Build history of the part. All positions in model axes, mm. A direction names the side the tool comes from. Round coordinates to 2 decimals unless told otherwise and drop trailing zeros. Write each loop counter-clockwise with the first axis right and the second up, starting at its lowest first coordinate (ties: lowest second). Pieces come first, ordered by that corner, then holes. Notation, with made-up numbers: (59.5, 39.25) - (93.5, 39.25) arc R14 cw to (93.5, 46.25) - close; hole circle Ø5 at (-20, 7.25). An arc over 180 degrees is marked (long way). One line per question, with ' | ' between items.
from build123d import *

# Parameters (mm, degrees)
SKETCH1_R           = 7.5565
SKETCH1_W           = 2.54
SKETCH1_H           = 4.572
BOSS_EXTRUDE1_DEPTH = 3.175


with BuildPart() as part:
    # Sketch1 → Boss-Extrude1 (new body)
    with BuildSketch(Plane.XY):
        with BuildLine():
            Line((-8.255, 15.639992312), (76.835, 15.639992312))
            ThreePointArc((76.835, 15.639992312), (80.876115254, 13.966107566), (82.55, 9.924992312))
            Line((82.55, 9.924992312), (82.55, -9.924992312))
            ThreePointArc((82.55, -9.924992312), (80.876115254, -13.966107566), (76.835, -15.639992312))
            Line((76.835, -15.639992312), (-8.255, -15.639992312))
            ThreePointArc((-8.255, -15.639992312), (-12.296115254, -13.966107566), (-13.97, -9.924992312))
            Line((-13.97, -9.924992312), (-13.97, 9.924992312))
            ThreePointArc((-13.97, 9.924992312), (-12.296115254, 13.966107566), (-8.255, 15.639992312))
        make_face()
        Circle(SKETCH1_R, mode=Mode.SUBTRACT)
        with Locations((22.86, 0)):
            Circle(SKETCH1_R, mode=Mode.SUBTRACT)
        with Locations((45.72, 0)):
            Circle(SKETCH1_R, mode=Mode.SUBTRACT)
        with Locations((68.58, 0)):
            Circle(SKETCH1_R, mode=Mode.SUBTRACT)
        with Locations((8.636, 12.083992312)):
            Rectangle(SKETCH1_W, SKETCH1_H, mode=Mode.SUBTRACT)
        with Locations((14.224, 12.083992312)):
            Rectangle(SKETCH1_W, SKETCH1_H, mode=Mode.SUBTRACT)
        with Locations((31.496, 12.083992312)):
            Rectangle(SKETCH1_W, SKETCH1_H, mode=Mode.SUBTRACT)
        with Locations((37.084, 12.083992312)):
            Rectangle(SKETCH1_W, SKETCH1_H, mode=Mode.SUBTRACT)
        with Locations((54.356, 12.083992312)):
            Rectangle(SKETCH1_W, SKETCH1_H, mode=Mode.SUBTRACT)
        with Locations((59.944, 12.083992312)):
            Rectangle(SKETCH1_W, SKETCH1_H, mode=Mode.SUBTRACT)
        with Locations((59.944, -12.083992312)):
            Rectangle(SKETCH1_W, SKETCH1_H, mode=Mode.SUBTRACT)
        with Locations((54.356, -12.083992312)):
            Rectangle(SKETCH1_W, SKETCH1_H, mode=Mode.SUBTRACT)
        with Locations((37.084, -12.083992312)):
            Rectangle(SKETCH1_W, SKETCH1_H, mode=Mode.SUBTRACT)
        with Locations((31.496, -12.083992312)):
            Rectangle(SKETCH1_W, SKETCH1_H, mode=Mode.SUBTRACT)
        with Locations((14.224, -12.083992312)):
            Rectangle(SKETCH1_W, SKETCH1_H, mode=Mode.SUBTRACT)
        with Locations((8.636, -12.083992312)):
            Rectangle(SKETCH1_W, SKETCH1_H, mode=Mode.SUBTRACT)
    extrude(amount=BOSS_EXTRUDE1_DEPTH)


solid = part.part
Q1. Saw through at A-A, the plane x = 45.72. List the corners of the cut face in (y, z) (1 decimal), then the cut area to 3 significant figures.
Found:
outline: (-15.6, 0) - (-7.6, 0) - (-7.6, 3.2) - (-15.6, 3.2) - close; (7.6, 0) - (15.6, 0) - (15.6, 3.2) - (7.6, 3.2) - close | area: 51.3 mm^2
Q2. Which spindle directions (+Z, -Z, +X, -X, +Y, -Y) get a long thin tool onto all of the face, cutting with end or side? Do faces 4 (the flat face through (35, 0, 3.175)), 5 (the flat face through (37, 14.37, 2)). Say none if no direction does.
Found:
face 4: +Z, +X, -X, +Y, -Y | face 5: +Z, -Z
Q3. Saw through at B-B, the plane y = 0. State how many separate pieces and enclosed holes the cut face has, then the cut area to 3 significant figures.
Found:
separate pieces: 5 | enclosed holes: 0 | area: 115 mm^2
Q4. Saw through at C-C, the plane y = 13. List the corners of the cut face in (x, z) (3 decimals).
Found:
outline: (-13.072, 0) - (7.366, 0) - (7.366, 3.175) - (-13.072, 3.175) - close; (9.906, 0) - (12.954, 0) - (12.954, 3.175) - (9.906, 3.175) - close; (15.494, 0) - (30.226, 0) - (30.226, 3.175) - (15.494, 3.175) - close; (32.766, 0) - (35.814, 0) - (35.814, 3.175) - (32.766, 3.175) - close; (38.354, 0) - (53.086, 0) - (53.086, 3.175) - (38.354, 3.175) - close; (55.626, 0) - (58.674, 0) - (58.674, 3.175) - (55.626, 3.175) - close; (61.214, 0) - (81.652, 0) - (81.652, 3.175) - (61.214, 3.175) - close
Q5. Drop flat-ended pins along their axis: pin 1 (1 mm diameter, centred on y = 11.5, z = 2.5, fed in from +X); pin 2 (13.5 mm diameter, centred on x = 0, y = 0, fed in from -Z); pin 3 (1 mm diameter, centred on y = -11.5, z = 1, fed in from -X). Give the stop position or say it passes through.
Found:
pin 1: x = 82.45 | pin 2: through | pin 3: x = -13.87
Q6. Pull direction X, two halves, no side cores. Call faces 1 (the flat face through (82.55, 0, 2)), 2 (the flat face through (54, -9.798, 2)), 3 (the cylindrical face through (-12.34, 13.92, 1.57)): +X half, -X half, draft (parallel to the pull), parting line (faces both ways), or undercut.
Found:
face 1: +X half | face 2: undercut | face 3: -X half
Q7. Drill centre lines: L1, parallel to Y at x = 59.5, z = 0.4; L2, parallel to Y at x = 22.86, z = 0.8; L3, parallel to X at y = -3.5, z = 1.35. Where is each one in solid material? Low to high. Write a range as from..to.
Found:
L1: -15.64..-14.37, -9.8..9.8, 14.37..15.64 | L2: -15.64..-7.56, 7.56..15.64 | L3: -13.97..-6.7, 6.7..16.16, 29.56..39.02, 52.42..61.88, 75.28..82.55
